```python
from build123d import *

# Parameters (mm, degrees)
SKETCH1_R           = 50
BOSS_EXTRUDE1_DEPTH = 13
FILLET1_R           = 6
FILLET2_R           = 6
SKETCH2_R           = 2
CUT_EXTRUDE1_DEPTH  = 13
CIRPATTERN1_COUNT   = 8


with BuildPart() as part:
    # Sketch1 → Boss-Extrude1 (new body)
    with BuildSketch(Plane(origin=(0, 0, 0), x_dir=(1, 0, 0), z_dir=(0, 1, 0))):
        with Locations(Location((0, 0, 0), (0, 0, 90))):
            Circle(SKETCH1_R)
        with BuildLine():
            ThreePointArc((36.323181231, 9.32075669), (36.779448015, 7.315887076), (37.125142857, 5.289023335))
            ThreePointArc((37.125142857, 5.289023335), (39.722463038, 3.191918366), (40.7, 0))
            ThreePointArc((40.7, 0), (39.722463038, -3.191918366), (37.125142857, -5.289023335))
            ThreePointArc((37.125142857, -5.289023335), (36.779448015, -7.315887076), (36.323181231, -9.32075669))
            ThreePointArc((36.323181231, -9.32075669), (37.590218254, -11.184640418), (38.035783638, -13.393920133))
            ThreePointArc((38.035783638, -13.393920133), (36.344793491, -17.445813517), (32.275138024, -19.093597502))
            ThreePointArc((32.275138024, -19.093597502), (31.180110461, -20.833883738), (29.991344533, -22.511536001))
            ThreePointArc((29.991344533, -22.511536001), (30.333218561, -23.606997658), (30.448737342, -24.748737342))
            ThreePointArc((30.448737342, -24.748737342), (27.890230009, -29.504893754), (22.511536001, -29.991344533))
            ThreePointArc((22.511536001, -29.991344533), (20.833883738, -31.180110461), (19.093597502, -32.275138024))
            ThreePointArc((19.093597502, -32.275138024), (19.093839474, -32.305460402), (19.093920133, -32.335783638))
            ThreePointArc((19.093920133, -32.335783638), (15.547169813, -37.613426655), (9.32075669, -36.323181231))
            ThreePointArc((9.32075669, -36.323181231), (7.315887076, -36.779448015), (5.289023335, -37.125142857))
            ThreePointArc((5.289023335, -37.125142857), (0, -40.7), (-5.289023335, -37.125142857))
            ThreePointArc((-5.289023335, -37.125142857), (-7.315887076, -36.779448015), (-9.32075669, -36.323181231))
            ThreePointArc((-9.32075669, -36.323181231), (-15.575215697, -37.601896973), (-19.093597502, -32.275138024))
            ThreePointArc((-19.093597502, -32.275138024), (-20.833883738, -31.180110461), (-22.511536001, -29.991344533))
            ThreePointArc((-22.511536001, -29.991344533), (-28.779245994, -28.779245994), (-29.991344533, -22.511536001))
            ThreePointArc((-29.991344533, -22.511536001), (-31.180110461, -20.833883738), (-32.275138024, -19.093597502))
            ThreePointArc((-32.275138024, -19.093597502), (-37.601896973, -15.575215697), (-36.323181231, -9.32075669))
            ThreePointArc((-36.323181231, -9.32075669), (-36.779448015, -7.315887076), (-37.125142857, -5.289023335))
            ThreePointArc((-37.125142857, -5.289023335), (-40.7, 0), (-37.125142857, 5.289023335))
            ThreePointArc((-37.125142857, 5.289023335), (-36.779448015, 7.315887076), (-36.323181231, 9.32075669))
            ThreePointArc((-36.323181231, 9.32075669), (-37.601896973, 15.575215697), (-32.275138024, 19.093597502))
            ThreePointArc((-32.275138024, 19.093597502), (-31.180110461, 20.833883738), (-29.991344533, 22.511536001))
            ThreePointArc((-29.991344533, 22.511536001), (-28.779245994, 28.779245994), (-22.511536001, 29.991344533))
            ThreePointArc((-22.511536001, 29.991344533), (-20.833883738, 31.180110461), (-19.093597502, 32.275138024))
            ThreePointArc((-19.093597502, 32.275138024), (-15.575215697, 37.601896973), (-9.32075669, 36.323181231))
            ThreePointArc((-9.32075669, 36.323181231), (-7.315887076, 36.779448015), (-5.289023335, 37.125142857))
            ThreePointArc((-5.289023335, 37.125142857), (0, 40.7), (5.289023335, 37.125142857))
            ThreePointArc((5.289023335, 37.125142857), (7.315887076, 36.779448015), (9.32075669, 36.323181231))
            ThreePointArc((9.32075669, 36.323181231), (15.547169813, 37.613426655), (19.093920133, 32.335783638))
            ThreePointArc((19.093920133, 32.335783638), (19.093839474, 32.305460402), (19.093597502, 32.275138024))
            ThreePointArc((19.093597502, 32.275138024), (20.833883738, 31.180110461), (22.511536001, 29.991344533))
            ThreePointArc((22.511536001, 29.991344533), (27.890230009, 29.504893754), (30.448737342, 24.748737342))
            ThreePointArc((30.448737342, 24.748737342), (30.333218561, 23.606997658), (29.991344533, 22.511536001))
            ThreePointArc((29.991344533, 22.511536001), (31.180110461, 20.833883738), (32.275138024, 19.093597502))
            ThreePointArc((32.275138024, 19.093597502), (36.344793491, 17.445813517), (38.035783638, 13.393920133))
            ThreePointArc((38.035783638, 13.393920133), (37.590218254, 11.184640418), (36.323181231, 9.32075669))
        make_face(mode=Mode.SUBTRACT)
    extrude(amount=BOSS_EXTRUDE1_DEPTH)

    # Fillet1
    # the kernel refuses this fillet: 6 mm, written as the material it takes off along each edge
    with BuildSketch(Plane(origin=(-19.093597502, -6.083636121, -32.275138024), x_dir=(0.14995847999359607, 0, -0.9886922950433115), z_dir=(0, 1, 0)), Plane(origin=(-29.991344533, -6.083636121, -22.511536001), x_dir=(-0.2398125906274579, 0, -0.9708192011783384), z_dir=(0, 1, 0)), Plane(origin=(-36.323181231, -6.083636121, -9.32075669), x_dir=(-0.5930743682320851, 0, -0.8051476844319388), z_dir=(0, 1, 0)), Plane(origin=(-37.125142857, -6.083636121, 5.289023335), x_dir=(-0.8560459495059065, 0, -0.5168997314127094), z_dir=(0, 1, 0)), Plane(origin=(-32.275138024, -6.083636121, 19.093597502), x_dir=(-0.988692295043333, 0, -0.14995847999345324), z_dir=(0, 1, 0)), Plane(origin=(-22.511536001, -6.083636121, 29.991344533), x_dir=(-0.9708192011784058, 0, 0.23981259062718507), z_dir=(0, 1, 0)), Plane(origin=(-9.32075669, -6.083636121, 36.323181231), x_dir=(-0.8051476844318383, 0, 0.5930743682322216), z_dir=(0, 1, 0)), Plane(origin=(5.289023335, -6.083636121, 37.125142857), x_dir=(-0.5168997314124754, 0, 0.8560459495060478), z_dir=(0, 1, 0)), Plane(origin=(29.991344533, -6.083636121, 22.511536001), x_dir=(0.2398125906274932, 0, 0.9708192011783298), z_dir=(0, 1, 0)), Plane(origin=(36.323181231, -6.083636121, 9.32075669), x_dir=(0.5930743682321865, 0, 0.8051476844318642), z_dir=(0, 1, 0)), Plane(origin=(37.125142857, -6.083636121, -5.289023335), x_dir=(0.8560459495059013, 0, 0.5168997314127179), z_dir=(0, 1, 0)), Plane(origin=(32.275138024, -6.083636121, -19.093597502), x_dir=(0.9886922950433297, 0, 0.14995847999347464), z_dir=(0, 1, 0)), Plane(origin=(9.32075669, -6.083636121, -36.323181231), x_dir=(0.8051476844318497, 0, -0.5930743682322063), z_dir=(0, 1, 0)), Plane(origin=(-5.289023335, -6.083636121, -37.125142857), x_dir=(0.5168997314124864, 0, -0.8560459495060411), z_dir=(0, 1, 0))) as fillet1_piece_1:
        with BuildLine():
            CenterArc((2.792165198, 5.922245026), FILLET1_R, 222.951284649, 37.814580314)
            ThreePointArc((-1.599434612, 1.833987316), (-0.784836973, 0.929970912), (0, 0))
            ThreePointArc((0, 0), (0.914674806, 0.073867225), (1.829349612, 0))
        make_face()
    extrude(amount=25.167272242, mode=Mode.SUBTRACT)
    with BuildSketch(Plane(origin=(-22.511536001, -6.083636121, -29.991344533), x_dir=(0.8188257163349287, 0, -0.5740421990312129), z_dir=(0, 1, 0)), Plane(origin=(-37.125142857, -6.083636121, -5.289023335), x_dir=(0.17308808500835637, 0, -0.9849063482525331), z_dir=(0, 1, 0)), Plane(origin=(-36.323181231, -6.083636121, 9.32075669), x_dir=(-0.21699480284666314, 0, -0.9761727590634447), z_dir=(0, 1, 0)), Plane(origin=(-29.991344533, -6.083636121, 22.511536001), x_dir=(-0.5740421990310322, 0, -0.8188257163350555), z_dir=(0, 1, 0)), Plane(origin=(-19.093597502, -6.083636121, 32.275138024), x_dir=(-0.8436968741184279, 0, -0.5368198809682758), z_dir=(0, 1, 0)), Plane(origin=(-5.289023335, -6.083636121, 37.125142857), x_dir=(-0.9849063482524983, 0, -0.17308808500855408), z_dir=(0, 1, 0)), Plane(origin=(22.511536001, -6.083636121, 29.991344533), x_dir=(-0.8188257163349197, 0, 0.574042199031226), z_dir=(0, 1, 0)), Plane(origin=(32.275138024, -6.083636121, 19.093597502), x_dir=(-0.5368198809683398, 0, 0.8436968741183872), z_dir=(0, 1, 0)), Plane(origin=(37.125142857, -6.083636121, 5.289023335), x_dir=(-0.17308808500835057, 0, 0.984906348252534), z_dir=(0, 1, 0)), Plane(origin=(36.323181231, -6.083636121, -9.32075669), x_dir=(0.21699480284658396, 0, 0.9761727590634621), z_dir=(0, 1, 0)), Plane(origin=(29.991344533, -6.083636121, -22.511536001), x_dir=(0.5740421990310425, 0, 0.8188257163350484), z_dir=(0, 1, 0)), Plane(origin=(19.093597502, -6.083636121, -32.275138024), x_dir=(0.8436968741184294, 0, 0.5368198809682734), z_dir=(0, 1, 0)), Plane(origin=(5.289023335, -6.083636121, -37.125142857), x_dir=(0.9849063482524999, 0, 0.17308808500854556), z_dir=(0, 1, 0)), Plane(origin=(-9.32075669, -6.083636121, -36.323181231), x_dir=(0.976172759063475, 0, -0.2169948028465263), z_dir=(0, 1, 0))) as fillet1_piece_2:
        with BuildLine():
            CenterArc((2.628130804, 5.996840928), FILLET1_R, 230.326071091, 37.814580314)
            ThreePointArc((-1.202375121, 1.378700139), (-0.54551709, 0.73790072), (0, 0))
            ThreePointArc((0, 0), (1.216727224, 0.0197442), (2.433454448, 0))
        make_face()
    extrude(amount=25.167272242, mode=Mode.SUBTRACT)
    with BuildSketch(Plane(origin=(9.32075669, -6.083636122, 36.323181231), x_dir=(-0.9761727590638747, 0, 0.2169948028447281), z_dir=(0, 1, 0))) as fillet1_piece_3:
        with BuildLine():
            CenterArc((2.628130805, 5.996840928), FILLET1_R, 230.326071091, 37.814580314)
            ThreePointArc((-1.202375121, 1.378700139), (-0.54551709, 0.73790072), (0, 0))
            ThreePointArc((0, 0), (1.216727224, 0.0197442), (2.433454449, 0))
        make_face()
    extrude(amount=25.167272243, mode=Mode.SUBTRACT)
    with BuildSketch(Plane(origin=(19.093597502, -6.083636121, 32.275138024), x_dir=(-0.14995847999251055, 0, 0.988692295043476), z_dir=(0, 1, 0))) as fillet1_piece_4:
        with BuildLine():
            CenterArc((2.792165198, 5.922245026), FILLET1_R, 222.951284649, 37.814580314)
            ThreePointArc((-1.599434612, 1.833987316), (-0.784836973, 0.929970912), (0, 0))
            ThreePointArc((0, 0), (0.914674806, 0.073867225), (1.829349613, 0))
        make_face()
    extrude(amount=25.167272242, mode=Mode.SUBTRACT)
    with BuildSketch(Plane(origin=(22.511536001, -6.083636121, -29.991344533), x_dir=(-0.81882571633492, 0, -0.5740421990312257), z_dir=(0, 1, 0))) as fillet1_piece_5:
        with BuildLine():
            CenterArc((2.628130804, -5.996840928), FILLET1_R, 91.859348595, 37.814580314)
            ThreePointArc((-1.202375121, -1.378700139), (-0.54551709, -0.73790072), (0, 0))
            ThreePointArc((0, 0), (1.216727224, -0.0197442), (2.433454448, 0))
        make_face()
    extrude(amount=25.167272242, mode=Mode.SUBTRACT)

    # Fillet2
    # the kernel refuses this fillet: 6 mm, written as the material it takes off along each edge
    with BuildSketch(Plane(origin=(-32.275138024, -4.443316345, -19.093597502), x_dir=(0.5282998062723766, 0, -0.8490578983158743), z_dir=(0, 1, 0))) as fillet2_piece_1:
        with BuildLine():
            CenterArc((2.770578985, 5.899824462), FILLET2_R, 229.219707945, 30.295762434)
            Line((-1.148382112, 1.35650586), (-1.226761334, 1.265639488))
            ThreePointArc((-1.226761334, 1.265639488), (-0.612581404, 0.645752673), (-0.102555687, -0.062308354))
            Line((-0.102555687, -0.062308354), (0.002686014, -0.119969935))
            ThreePointArc((0.002686014, -0.119969935), (0.839379399, -0.110604719), (1.656922395, -0.117996489))
            Line((1.656922395, -0.117996489), (1.678758799, 0))
        make_face()
    extrude(amount=21.88663269, mode=Mode.SUBTRACT)

    # Sketch2 → Cut-Extrude1 (cut)
    with BuildSketch(Plane(origin=(0, 13, 0), x_dir=(1, 0, 0), z_dir=(0, 1, 0))):
        with Locations(Location((37.416132554, 25.000660486, 0), (0, 0, 270))):
            Circle(SKETCH2_R)
    cut_extrude1 = extrude(amount=-CUT_EXTRUDE1_DEPTH, mode=Mode.SUBTRACT)

    # CirPattern1: Cut-Extrude1 ×8 about axis
    cirpattern1_axis = Axis((0, 0, 0), (0, 1, 0))
    for i in range(1, CIRPATTERN1_COUNT):
        add(cut_extrude1.rotate(cirpattern1_axis, i * 360 / CIRPATTERN1_COUNT), mode=Mode.SUBTRACT)


solid = part.part
```
Can you work these out from the model? Positions are in its coordinate system, mm. Give positions to 0.01 mm unless a question says otherwise; leave off trailing zeros. Order: outer loops, then holes, each group sorted by start corner. A loop starts at its lowest first (then second) coordinate and runs counter-clockwise, first axis right, second up. Notation, with made-up numbers: M 37.5,49 L 68.5,49 A26 cw 68.5,67 Z; hole C -16,-13 d2. An arc over 180 degrees is marked long. Write item = value, one per line. Start each with the question number.
Q1. We'd pull the mould along Z, two halves only. Please class faces 1 (the cylindrical face through (19.627, 6.409, 32.465)), 2 (the flat face through (37, 13, 8)): pulls with the +Z half, pulls with the -Z half, needs draft (parallel to the pull), parting line crosses it, or undercut.
Q2. Suppose I cut it at B-B (z = -29). Write out the boundary of the cut face in (x, y).
Q3. Suppose I cut it at A-A (x = 0). Write out the boundary of the cut face in (y, z), plus the area to 3 significant figures.
Q4. Suppose I cut it at C-C (y = 8.75). Count the separate pieces of the cut face and the enclosed holes in it, plus the area to 3 significant figures.
Q5. I need wall thicknesses on probe 1 along X at (y, z) = (7.5, 7.5); probe 2 along X at (y, z) = (3.5, -9.5); probe 3 along Z at (x, y) = (7.5, 2). Which ranges of each line are inside material? Lowest first, please. Write a range as [from, to].
Q6. Will these pins go through, and if not, where does the flat tip stop? pin 1 Ø4.5 at (x, z) = (8.78, -44.14) entering from -Y; pin 2 Ø4 at (y, z) = (7, 5.5) entering from +X; pin 3 Ø2 at (y, z) = (11.5, -18) entering from +X; pin 4 Ø4 at (x, y) = (4.5, 9.5) entering from -Z.
Check result:
q1.face_1 = undercut
q1.face_2 = needs draft
q2.outline = M -40.73,0 L -28.55,0 L -28.55,13 L -40.73,13 Z; M 28.55,0 L 40.73,0 L 40.73,13 L 28.55,13 Z
q3.outline = M 0,-50 L 13,-50 L 13,-40.7 L 0,-40.7 Z; M 0,40.7 L 13,40.7 L 13,50 L 0,50 Z
q3.area = 242 mm2
q4.separate_pieces = 1
q4.enclosed_holes = 9
q4.area = 2,920 mm2
q5.probe_1 = [-49.43, -36.77], [36.77, 42.6], [45.67, 49.43]
q5.probe_2 = [-49.09, -46], [-42.27, -36.92], [36.92, 49.09]
q5.probe_3 = [-49.43, -45.67], [-42.6, -36.77], [36.77, 49.43]
q6.pin_1 = 0
q6.pin_2 = 49.88
q6.pin_3 = 47.02
q6.pin_4 = -49.94
